Study the drawing (mm; zero at the part's minimum x, y, z) and answer. A direction names the side the tool comes from. Give positions to 0.01 mm unless a question says otherwise; leave off trailing zeros. Loops run counter-clockwise (first coordinate to the right, second up) from the corner with the lowest first, then second, coordinate; pieces in that order, holes last. Notation, with made-up numbers: (38, -2.5) - (71, -2.5) arc R27 ccw to (71, 20.5) - close; hole circle Ø10 at (12.5, 50). An arc over 180 degrees is marked (long way). Write item = value, one per line. Start each with the question number.
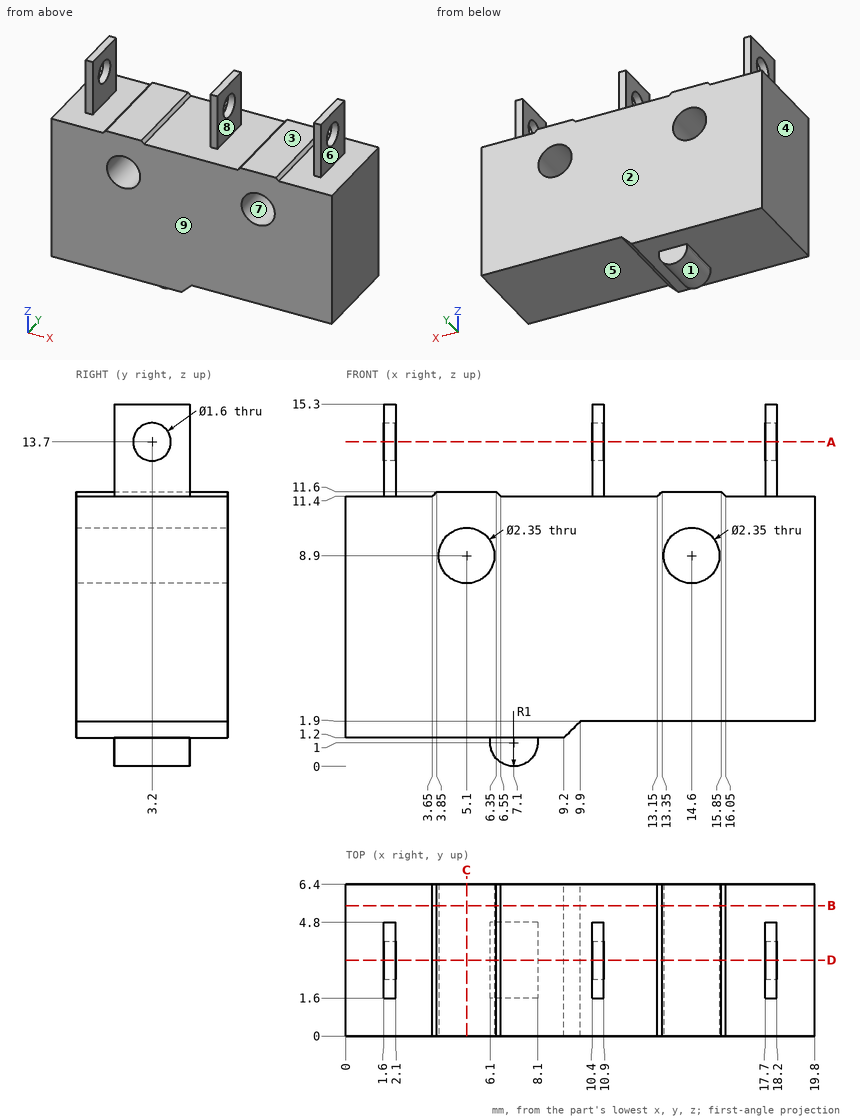
1. For a pull along X with two mould halves and no side action, classify the marked faces 1, 2, 3 and 4 as released by +X, released by -X, zero draft, split by the parting line, or undercut.
2. A cutting plane is placed at D-D on y = 3.2. Give the number of separate pieces and of enclosed holes in the cut face, and give its area (3 significant figures).
3. Given P1, Ø2, axis at x = 5.5, y = 3, coming from the +Z side; P2, Ø1, axis at x = 6, z = 13.5, coming from the -Y side; P3, Ø3.5, axis at y = 3.5, z = 13, coming from the -X side; P4, Ø1.3, axis at x = 7.5, z = 0.5, coming from the -Y side, each flat-ended and moving along its own axis, determine where each tip first touches the part or whether it passes through.
4. A cutting plane is placed at A-A on z = 13.7. Give the vertices of the cut face in (x, y).
5. Consider line 1 along X through (y, z) = (4, 12.25); line 2 along X through (y, z) = (2.25, 8.9) (3 decimals); line 3 along Y through (x, z) = (1.95, 13.7). Determine where each line is inside the solid, lowest interval first. Write a range as [from, to].
6. A tool of negligible diameter and unlimited length cuts with its end or side. For the marked faces 5, 6, 7, 8 and 9, from which of +Z, -Z, +X, -X, +Y, -Y can it reach the whole face along a straight path? Write none if from no direction.
7. A cutting plane is placed at C-C on x = 5.1. Give the vertices of the cut face in (y, z) (3 decimals), and give its area (3 significant figures).
8. A cutting plane is placed at B-B on y = 5.5. Give the vertices of the cut face in (x, z) (3 decimals), and give its area (3 significant figures).
Reply:
q1.face_1 = split by the parting line
q1.face_2 = zero draft
q1.face_3 = undercut
q1.face_4 = released by -X
q2.separate_pieces = 4
q2.enclosed_holes = 2
q2.area = 193 mm^2
q3.P1 = 11.6
q3.P2 = through
q3.P3 = 0
q3.P4 = 1.6
q4.outline = (1.6, 1.6) - (2.1, 1.6) - (2.1, 2.4) - (1.6, 2.4) - close; (1.6, 4) - (2.1, 4) - (2.1, 4.8) - (1.6, 4.8) - close; (10.4, 1.6) - (10.9, 1.6) - (10.9, 2.4) - (10.4, 2.4) - close; (10.4, 4) - (10.9, 4) - (10.9, 4.8) - (10.4, 4.8) - close; (17.7, 1.6) - (18.2, 1.6) - (18.2, 2.4) - (17.7, 2.4) - close; (17.7, 4) - (18.2, 4) - (18.2, 4.8) - (17.7, 4.8) - close
q5.line_1 = [1.6, 2.1], [10.4, 10.9], [17.7, 18.2]
q5.line_2 = [0, 3.925], [6.275, 13.425], [15.775, 19.8]
q5.line_3 = [1.6, 2.4], [4, 4.8]
q6.face_5 = -Z, +X, +Y, -Y
q6.face_6 = +Z, +X, +Y, -Y
q6.face_7 = +Y, -Y
q6.face_8 = +Z, +Y, -Y
q6.face_9 = +Z, -Z, +X, -X, -Y
q7.outline = (0, 1.2) - (6.4, 1.2) - (6.4, 7.725) - (0, 7.725) - close; (0, 10.075) - (6.4, 10.075) - (6.4, 11.6) - (0, 11.6) - close
q7.area = 51.5 mm^2
q8.outline = (0, 1.2) - (9.2, 1.2) - (9.9, 1.9) - (19.8, 1.9) - (19.8, 11.4) - (16.05, 11.4) - (15.85, 11.6) - (13.35, 11.6) - (13.15, 11.4) - (6.55, 11.4) - (6.35, 11.6) - (3.85, 11.6) - (3.65, 11.4) - (0, 11.4) - close; hole circle Ø2.35 at (5.1, 8.9); hole circle Ø2.35 at (14.6, 8.9)
q8.area = 187 mm^2
